Can you work these out from the drawing? Everything is in mm from the part's minimum corner. A direction names the side the tool comes from. Round coordinates to 2 decimals unless told otherwise and drop trailing zeros. Loops run counter-clockwise (first coordinate to the right, second up) from the corner with the lowest first, then second, coordinate; pieces in that order, holes last. Notation, with made-up numbers: M 75.5,1.5 L 124.5,1.5 A6 cw 124.5,5.5 Z; hole C -20.5,31.5 d10. An arc over 180 degrees is marked long. One line per question, with ' | ' between items. Start each with the question number.
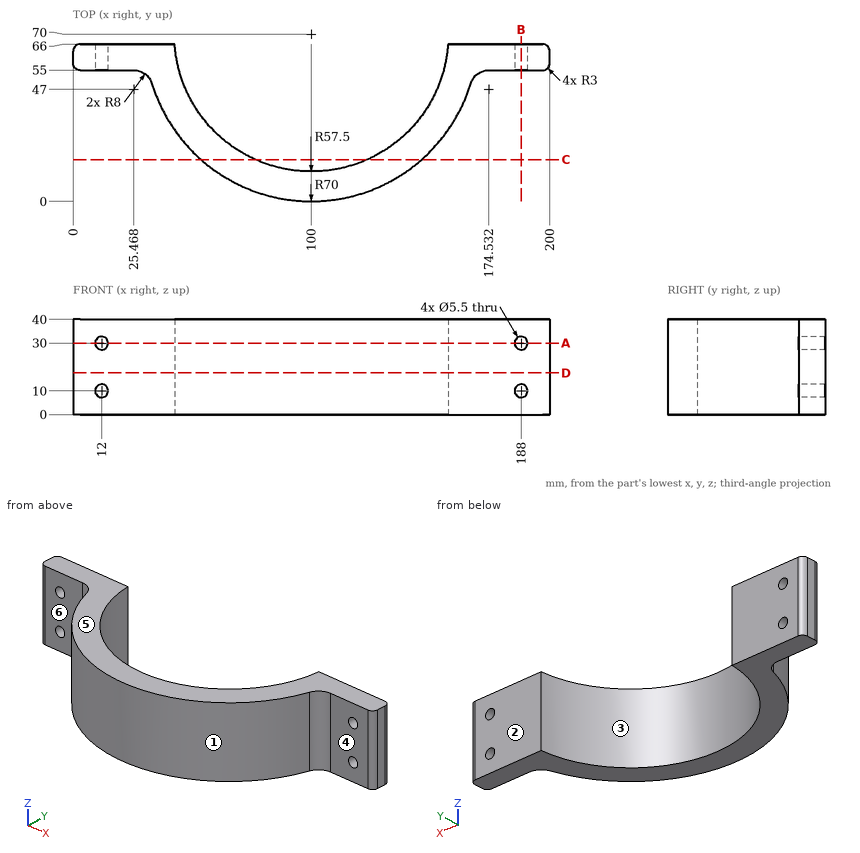
1) Imagine slicing it at A-A (z = 30). Write out the boundary of the cut face in (x, y), then the cut area to 3 significant figures.
2) Please list where these lines run through material, in increasing order: L1, parallel to Z at x = 188, y = 62; L2, parallel to Y at x = 21.5, z = 21; L3, parallel to X at y = 16.5, z = 16. Write a range as from..to.
3) Imagine slicing it at D-D (z = 17.5). Write out the boundary of the cut face in (x, y).
4) For the marked faces 4, 5 and 6, which set-ups out of +Z, -Z, +X, -X, +Y, -Y let a thin tool reach every point of the face, with its end or its side?
5) Imagine slicing it at C-C (y = 17.5). Write out the boundary of the cut face in (x, z).
6) I'm going to push flat-ended pins straight in: pin 1 Ø10 at (y, z) = (9, 12) entering from -X; pin 2 Ø1.5 at (y, z) = (26, 34) entering from +X; pin 3 Ø12 at (x, z) = (30.5, 31.5) entering from -Y. Where does each tip first touch, or does it pass through?
7) We'd pull the mould along X, two halves only. Please class the marked faces 1, 2 and 3: pulls with the +X half, pulls with the -X half, needs draft (parallel to the pull), parting line crosses it, or undercut.
8) Imagine slicing it at B-B (x = 188). Write out the boundary of the cut face in (y, z).
Results are:
1) outline: M 0,58 A3 ccw 3,55 L 9.25,55 L 9.25,66 L 3,66 A3 ccw 0,63 Z; M 14.75,55 L 25.47,55 A8 cw 33.11,49.36 A70 ccw 166.89,49.36 A8 cw 174.53,55 L 185.25,55 L 185.25,66 L 157.36,66 A57.5 cw 42.64,66 L 14.75,66 Z; M 190.75,55 L 197,55 A3 ccw 200,58 L 200,63 A3 ccw 197,66 L 190.75,66 Z | area: 2,960 mm²
2) L1: 0..7.25, 12.75..27.25, 32.75..40 | L2: 55..66 | L3: 54.86..78.93, 121.07..145.14
3) outline: M 0,58 A3 ccw 3,55 L 25.47,55 A8 cw 33.11,49.36 A70 ccw 166.89,49.36 A8 cw 174.53,55 L 197,55 A3 ccw 200,58 L 200,63 A3 ccw 197,66 L 157.36,66 A57.5 cw 42.64,66 L 3,66 A3 ccw 0,63 Z
4) face 4: +Z, -Z, +X, -Y | face 5: +Z, +X, -X, +Y, -Y | face 6: +Z, -Z, -X, -Y
5) outline: M 53.7,0 L 76.55,0 L 76.55,40 L 53.7,40 Z; M 123.45,0 L 146.3,0 L 146.3,40 L 123.45,40 Z
6) pin 1: x = 58 | pin 2: x = 155.04 | pin 3: y = 40.54
7) face 1: parting line crosses it | face 2: needs draft | face 3: undercut
8) outline: M 55,0 L 66,0 L 66,7.25 L 55,7.25 Z; M 55,12.75 L 66,12.75 L 66,27.25 L 55,27.25 Z; M 55,32.75 L 66,32.75 L 66,40 L 55,40 Z
